from build123d import *

# Parameters (mm, degrees)
F0_R     = 76.2
F0_W     = 25.4
F0_H     = 22.86
F1_DEPTH = 7.62
F3_T     = -2.54


# Not quite as in the source:
# - the program builds the solid bodies; features that only make, move or delete a surface that nothing else refers to are left out


with BuildPart() as f1:
    # F0 (on Front) → F1 (new body)
    with BuildSketch(Plane.XZ):
        with Locations((40.9205045223, 25.0884863067)):
            Circle(F0_R)
        with Locations((40.9205045223, 25.0884863067)):
            Rectangle(F0_W, F0_H, mode=Mode.SUBTRACT)
    extrude(amount=F1_DEPTH)

    # F3
    f3_openings = [f1.faces().sort_by_distance(p)[0] for p in [
        (-33.124234, -7.62, 25.088486),
    ]]
    offset(amount=F3_T, openings=f3_openings, kind=Kind.INTERSECTION)


solid = f1.part
Model file for the job. Use its own axes, mm. A direction names the side the tool comes from. Coordinates: 2 decimals unless noted, no trailing zeros. Loops run counter-clockwise (first coordinate to the right, second up) from the corner with the lowest first, then second, coordinate; pieces in that order, holes last. Notation, with made-up numbers: (-17, -4) -> (11, -4) arc R31 cw to (11, 26) -> close; hole circle Ø5 at (61.5, 63). An arc over 180 degrees is marked (long way). Use one line per item in the form item = value. Start each with the question number.
(1) Cut at D-D on x = 38. Give the cut face in (y, z), and give its area (3 significant figures).
(2) Tool access for faces 4 (the flat face through (41, -5, 11.118)), 5 (the flat face through (41, -7.62, 38)), 6 (the flat face through (28.221, -4, 25)): list every direction of +Z, -Z, +X, -X, +Y, -Y with a clear straight run to the whole face (end or side of a thin tool).
(3) Cut at A-A on y = -5. Give the cut face in (x, z).
(4) Probe probe 1 along Z at (x, y) = (39.5, -4.75); probe 2 along Z at (x, y) = (-19.5, -3.25); probe 3 along X at (y, z) = (-5, -8). List the from-to ranges inside material, lowest first. Write a range as from..to.
(5) Flat gauge pins, fed straight in: pin 1 (8 mm diameter, centred on x = 80, z = 47, fed in from +Y); pin 2 (6 mm diameter, centred on x = 58.5, z = -21.5, fed in from -Y); pin 3 (4 mm diameter, centred on x = 36.5, y = -2, fed in from +Z); pin 4 (1 mm diameter, centred on x = 34.5, y = -2.5, fed in from -Z). Where does each tip first touch, or does it go through?
(6) Pull direction X, two halves, no side cores. Call faces 1 (the cylindrical face through (24.4, -3.8, -49.3)), 2 (the flat face through (25.681, -5, 25)), 3 (the flat face through (1, -7.62, 88)): pulls with the +X half, pulls with the -X half, needs draft (parallel to the pull), parting line crosses it, or undercut.
(7) Cut at B-B on z = 29.5. Give the cut face in (x, y), and give its area (3 significant figures).
(8) Cut at C-C on x = 1.5. Give the cut face in (y, z).
Values:
q1.outline = (-7.62, -51.06) -> (0, -51.06) -> (0, 13.66) -> (-7.62, 13.66) -> (-7.62, 11.12) -> (-2.54, 11.12) -> (-2.54, -48.51) -> (-7.62, -48.51) -> close; (-7.62, 36.52) -> (0, 36.52) -> (0, 101.23) -> (-7.62, 101.23) -> (-7.62, 98.69) -> (-2.54, 98.69) -> (-2.54, 39.06) -> (-7.62, 39.06) -> close
q1.area = 380 mm2
q2.face_4 = -Y
q2.face_5 = +Z, -Z, +X, -X, -Y
q2.face_6 = +Y, -Y
q3.outline = circle Ø152.4 at (40.92, 25.09); (25.68, 11.12) -> (56.16, 11.12) -> (56.16, 39.06) -> (25.68, 39.06) -> close; hole circle Ø147.32 at (40.92, 25.09); hole (28.22, 13.66) -> (53.62, 13.66) -> (53.62, 36.52) -> (28.22, 36.52) -> close
q4.probe_1 = -51.1..-48.56, 11.12..13.66, 36.52..39.06, 98.73..101.28
q4.probe_2 = -21.34..-17.04, 67.22..71.52
q4.probe_3 = -27.72..-24.89, 106.73..109.56
q5.pin_1 = 0
q5.pin_2 = -2.54
q5.pin_3 = 101.25
q5.pin_4 = -50.88
q6.face_1 = parting line crosses it
q6.face_2 = undercut
q6.face_3 = needs draft
q7.outline = (-35.15, -7.62) -> (-32.61, -7.62) -> (-32.61, -2.54) -> (25.68, -2.54) -> (25.68, -7.62) -> (28.22, -7.62) -> (28.22, 0) -> (-35.15, 0) -> close; (53.62, -7.62) -> (56.16, -7.62) -> (56.16, -2.54) -> (114.45, -2.54) -> (114.45, -7.62) -> (116.99, -7.62) -> (116.99, 0) -> (53.62, 0) -> close
q7.area = 374 mm2
q8.outline = (-7.62, -40.12) -> (0, -40.12) -> (0, 90.3) -> (-7.62, 90.3) -> (-7.62, 87.31) -> (-2.54, 87.31) -> (-2.54, -37.14) -> (-7.62, -37.14) -> close
